Verification items for the finished model (mm, model axes). A direction names the side the tool comes from. Round coordinates to 2 decimals unless told otherwise and drop trailing zeros. Order: outer loops, then holes, each group sorted by start corner. A loop starts at its lowest first (then second) coordinate and runs counter-clockwise, first axis right, second up. Notation, with made-up numbers: (6, 5.5) -> (21, 5.5) arc R12 ccw to (21, 24.5) -> close; hole circle Ø11 at (47, 8). An arc over 180 degrees is marked (long way). Return JSON: item names as keys, results as strings. Group by question number.
1) Section check A-A on x = 299.5. Enter the section's corners in (y, z).
2) Tool access check on faces 1 (the flat face through (611, 37, -25)), 2 (the flat face through (611, 55, -250)), 3 (the flat face through (612, 10, -65)). Record the directions out of +Z, -Z, +X, -X, +Y, -Y that give a thin tool (end or side, any length) a straight path to the whole face; none if there is none.
3) Section check B-B on z = -98. Enter the section's corners in (x, y), plus the area to 3 significant figures.
4) Scan lines: L1, parallel to Z at x = 1100, y = 52; L2, parallel to Z at x = 1114, y = 44; L3, parallel to X at y = 4.5, z = -89.5. Record each from-to range of solid material in increasing order.
5) Depth check by flat-ended pin: pin 1 (3 mm diameter, centred on x = 619, z = -249, fed in from +Y); pin 2 (1.5 mm diameter, centred on y = 21, z = -139, fed in from -X). Enter the tip coordinate at first touch or a pass-through.
6) Draft check along Z on faces 4 (the flat face through (611, 20, -62)), 5 (the flat face through (611, 27, -262)), 6 (the flat face through (611, 0, -46)). Enter one of: pulls with the +Z half, pulls with the -Z half, needs draft (parallel to the pull), parting line crosses it, or undercut.
7) Section check C-C on y = 11.5. Enter the section's corners in (x, z).
```python
from build123d import *

# Parameters (mm, degrees)
SKETCH1_W           = 1240
SKETCH1_H           = 262
BOSS_EXTRUDE1_DEPTH = 20
SKETCH2_W           = 1240
SKETCH2_H           = 25
BOSS_EXTRUDE2_DEPTH = 35
SKETCH3_R           = 3
CUT_EXTRUDE1_DEPTH  = 10
SKETCH4_R           = 3
CUT_EXTRUDE2_DEPTH  = 10
SKETCH5_W           = 1160
SKETCH5_H           = 132
CUT_EXTRUDE3_DEPTH  = 21


with BuildPart() as part:
    # Sketch1 → Boss-Extrude1 (new body)
    with BuildSketch(Plane(origin=(0, 0, 0), x_dir=(1, 0, 0), z_dir=(0, 1, 0))):
        with Locations((620, 131)):
            Rectangle(SKETCH1_W, SKETCH1_H)
    extrude(amount=BOSS_EXTRUDE1_DEPTH)

    # Sketch2 → Boss-Extrude2 (add)
    with BuildSketch(Plane(origin=(0, 20, 0), x_dir=(1, 0, 0), z_dir=(0, 1, 0))):
        with Locations((620, 12.5)):
            Rectangle(SKETCH2_W, SKETCH2_H)
        with Locations((620, 249.5)):
            Rectangle(SKETCH2_W, SKETCH2_H)
    extrude(amount=BOSS_EXTRUDE2_DEPTH)

    # Sketch3 → Cut-Extrude1 (cut)
    with BuildSketch(Plane(origin=(0, 55, 0), x_dir=(1, 0, 0), z_dir=(0, 1, 0))):
        with Locations((20, 12.5)):
            Circle(SKETCH3_R)
        with Locations((80, 12.5)):
            Circle(SKETCH3_R)
        with Locations((140, 12.5)):
            Circle(SKETCH3_R)
        with Locations((200, 12.5)):
            Circle(SKETCH3_R)
        with Locations((260, 12.5)):
            Circle(SKETCH3_R)
        with Locations((320, 12.5)):
            Circle(SKETCH3_R)
        with Locations((380, 12.5)):
            Circle(SKETCH3_R)
        with Locations((440, 12.5)):
            Circle(SKETCH3_R)
        with Locations((500, 12.5)):
            Circle(SKETCH3_R)
        with Locations((560, 12.5)):
            Circle(SKETCH3_R)
        with Locations((620, 12.5)):
            Circle(SKETCH3_R)
        with Locations((680, 12.5)):
            Circle(SKETCH3_R)
        with Locations((740, 12.5)):
            Circle(SKETCH3_R)
        with Locations((800, 12.5)):
            Circle(SKETCH3_R)
        with Locations((860, 12.5)):
            Circle(SKETCH3_R)
        with Locations((920, 12.5)):
            Circle(SKETCH3_R)
        with Locations((980, 12.5)):
            Circle(SKETCH3_R)
        with Locations((1040, 12.5)):
            Circle(SKETCH3_R)
        with Locations((1100, 12.5)):
            Circle(SKETCH3_R)
        with Locations((1160, 12.5)):
            Circle(SKETCH3_R)
        with Locations((1220, 12.5)):
            Circle(SKETCH3_R)
    extrude(amount=-CUT_EXTRUDE1_DEPTH, mode=Mode.SUBTRACT)

    # Sketch4 → Cut-Extrude2 (cut)
    with BuildSketch(Plane(origin=(0, 55, 0), x_dir=(1, 0, 0), z_dir=(0, 1, 0))):
        with Locations((20, 249.5)):
            Circle(SKETCH4_R)
        with Locations((80, 249.5)):
            Circle(SKETCH4_R)
        with Locations((140, 249.5)):
            Circle(SKETCH4_R)
        with Locations((200, 249.5)):
            Circle(SKETCH4_R)
        with Locations((260, 249.5)):
            Circle(SKETCH4_R)
        with Locations((320, 249.5)):
            Circle(SKETCH4_R)
        with Locations((380, 249.5)):
            Circle(SKETCH4_R)
        with Locations((440, 249.5)):
            Circle(SKETCH4_R)
        with Locations((500, 249.5)):
            Circle(SKETCH4_R)
        with Locations((560, 249.5)):
            Circle(SKETCH4_R)
        with Locations((620, 249.5)):
            Circle(SKETCH4_R)
        with Locations((680, 249.5)):
            Circle(SKETCH4_R)
        with Locations((740, 249.5)):
            Circle(SKETCH4_R)
        with Locations((800, 249.5)):
            Circle(SKETCH4_R)
        with Locations((860, 249.5)):
            Circle(SKETCH4_R)
        with Locations((920, 249.5)):
            Circle(SKETCH4_R)
        with Locations((980, 249.5)):
            Circle(SKETCH4_R)
        with Locations((1040, 249.5)):
            Circle(SKETCH4_R)
        with Locations((1100, 249.5)):
            Circle(SKETCH4_R)
        with Locations((1160, 249.5)):
            Circle(SKETCH4_R)
        with Locations((1220, 249.5)):
            Circle(SKETCH4_R)
    extrude(amount=-CUT_EXTRUDE2_DEPTH, mode=Mode.SUBTRACT)

    # Sketch5 → Cut-Extrude3 (cut, through all)
    with BuildSketch(Plane(origin=(0, 20, 0), x_dir=(1, 0, 0), z_dir=(0, 1, 0))):
        with Locations((620, 131)):
            Rectangle(SKETCH5_W, SKETCH5_H)
    extrude(amount=-CUT_EXTRUDE3_DEPTH, mode=Mode.SUBTRACT)


solid = part.part
```
Check result:
{
 "1": {"outline": "(0, -262) -> (55, -262) -> (55, -237) -> (20, -237) -> (20, -197) -> (0, -197) -> close; (0, -65) -> (20, -65) -> (20, -25) -> (55, -25) -> (55, 0) -> (0, 0) -> close"},
 "2": {"face 1": "+X, -X, +Y", "face 2": "+Z, -Z, +X, -X, +Y", "face 3": "+Y, -Y"},
 "3": {"outline": "(0, 0) -> (40, 0) -> (40, 20) -> (0, 20) -> close; (1200, 0) -> (1240, 0) -> (1240, 20) -> (1200, 20) -> close", "area": "1,600 mm^2"},
 "4": {"L1": "-262 to -252.5, -246.5 to -237, -25 to -15.5, -9.5 to 0", "L2": "-262 to -237, -25 to 0", "L3": "0 to 40, 1200 to 1240"},
 "5": {"pin 1": "y = 45", "pin 2": "through"},
 "6": {"face 4": "undercut", "face 5": "pulls with the -Z half", "face 6": "needs draft"},
 "7": {"outline": "(0, -262) -> (1240, -262) -> (1240, 0) -> (0, 0) -> close; hole (40, -197) -> (1200, -197) -> (1200, -65) -> (40, -65) -> close"}
}
